from build123d import *

# Parameters (mm, degrees)
SKETCH1_W           = 100
SKETCH1_H           = 100
SKETCH1_R           = 2.5
BOSS_EXTRUDE1_DEPTH = 6
FILLET1_R           = 3


with BuildPart() as part:
    # Sketch1 → Boss-Extrude1 (new body)
    with BuildSketch(Plane(origin=(0, 0, 0), x_dir=(1, 0, 0), z_dir=(0, 1, 0))):
        with Locations((40, -40)):
            Rectangle(SKETCH1_W, SKETCH1_H)
        Circle(SKETCH1_R, mode=Mode.SUBTRACT)
        with Locations((80, 0)):
            Circle(SKETCH1_R, mode=Mode.SUBTRACT)
        with Locations((80, -80)):
            Circle(SKETCH1_R, mode=Mode.SUBTRACT)
        with Locations((0, -80)):
            Circle(SKETCH1_R, mode=Mode.SUBTRACT)
    extrude(amount=BOSS_EXTRUDE1_DEPTH)

    # Fillet1
    fillet1_edges = [part.edges().sort_by_distance(p)[0] for p in [
        (-10, 3, -10),
        (90, 3, -10),
        (90, 3, 90),
        (-10, 3, 90),
    ]]
    fillet(fillet1_edges, radius=FILLET1_R)


solid = part.part
Design review of the part built by this model. Coordinates are the model's own, in mm. Round coordinates to 2 decimals unless told otherwise and drop trailing zeros. Write each loop counter-clockwise with the first axis right and the second up, starting at its lowest first coordinate (ties: lowest second). Pieces come first, ordered by that corner, then holes. Notation, with made-up numbers: (-4, -12.5) - (54, -12.5) arc R12 ccw to (54, -3.5) - close; hole circle Ø4 at (41, -19). An arc over 180 degrees is marked (long way). Return JSON: item names as keys, results as strings. Group by question number.
Item 1: The part is to be moulded in two halves that separate along X. For faces 1 (the face through (90, 3, 41)), 2 (the face through (77.5, 3, 79.9)), 3 (the face through (39, 6, 39)), 4 (the face through (1.15, 2.96, 82.22)), say which applies: pulls with the +X half, pulls with the -X half, needs draft (parallel to the pull), parting line crosses it, or undercut.
Item 2: We need section A-A on x = 80. Write out the cut boundary in (y, z).
Item 3: For probe 1 along Z at (x, y) = (80, 1.7); probe 2 along X at (y, z) = (3.85, 2), list the stretches that pass through material, from the lowest coordinate up. Write a range as [from, to].
Item 4: We need section B-B on z = 80. Write out the cut boundary in (x, y), and give its area (3 significant figures).
Model answer:
{
 "1": {"face 1": "pulls with the +X half", "face 2": "undercut", "face 3": "needs draft", "face 4": "undercut"},
 "2": {"outline": "(0, -10) - (6, -10) - (6, -2.5) - (0, -2.5) - close; (0, 2.5) - (6, 2.5) - (6, 77.5) - (0, 77.5) - close; (0, 82.5) - (6, 82.5) - (6, 90) - (0, 90) - close"},
 "3": {"probe 1": "z = [-10, -2.5], [2.5, 77.5], [82.5, 90]", "probe 2": "x = [-10, -1.5], [1.5, 78.5], [81.5, 90]"},
 "4": {"outline": "(-10, 0) - (-2.5, 0) - (-2.5, 6) - (-10, 6) - close; (2.5, 0) - (77.5, 0) - (77.5, 6) - (2.5, 6) - close; (82.5, 0) - (90, 0) - (90, 6) - (82.5, 6) - close", "area": "540 mm²"}
}
